Source: CAD feature listing. Evaluate the final solid. Frame: model axes, mm. Face numbers are marked on the shaded views. A direction names the side the tool comes from. Coordinates: 2 decimals unless noted, no trailing zeros. Loops run counter-clockwise (first coordinate to the right, second up) from the corner with the lowest first, then second, coordinate; pieces in that order, holes last.
Item 1: Pull-direction query (Y, two-part tool) for the marked faces 4, 5, 6 and 7; classes: +Y half, -Y half, draft (parallel to the pull), parting line (faces both ways), or undercut.
Item 2: Section query C-C, the plane z = 7. Return the cut outline in (x, y), then the cut area to 3 significant figures.
Item 3: Section query A-A, the plane x = -26.5. Return the cut outline in (y, z).
Item 4: Section query D-D, the plane x = 8. Return the cut outline in (y, z), then the cut area to 4 significant figures.
Item 5: Pin query (flat end, axial travel): pin 1 Ø3 at (x, y) = (9.5, -18.5) entering from -Z; pin 2 Ø2 at (x, y) = (28, 18.5) entering from +Z. Return the tip coordinate at first contact, or that it passes through.
Item 6: Reachability of the marked faces 1, 2 and 3 from +Z, -Z, +X, -X, +Y, -Y: full face, straight path, thin tool, end or side. Return the list, or none.
Item 7: Line query: probe 1 along Y at (x, z) = (-1.5, 12); probe 2 along X at (y, z) = (29, 7); probe 3 along X at (y, z) = (8, 6.5). Output: solid intervals per line, ascending.
Item 8: Section query B-B, the plane y = -19.5. Return the cut outline in (x, z), then the cut area to 3 significant figures.
```python
from build123d import *

# Parameters (mm, degrees)
F0_W     = 70
F0_H     = 69
F1_DEPTH = 13
F2_W     = 59.5
F2_H     = 41.5
F3_DEPTH = 8
F4_W     = 16
F4_H     = 13.75
F5_DEPTH = 13.001
F7_DEPTH = 13.001


with BuildPart() as f1:
    # F0 (on Top) → F1 (new body)
    with BuildSketch(Plane.XY):
        Rectangle(F0_W, F0_H)
    extrude(amount=F1_DEPTH)

    # F2 (on face) → F3 (cut)
    with BuildSketch(Plane.XY.offset(13)):
        Rectangle(F2_W, F2_H)
    extrude(amount=-F3_DEPTH, mode=Mode.SUBTRACT)

    # F4 (on face) → F5 (cut, through all)
    with BuildSketch(Plane.XY.offset(13)):
        with Locations((17.75, 27.625)):
            Rectangle(F4_W, F4_H)
    extrude(amount=-F5_DEPTH, mode=Mode.SUBTRACT)

    # F6 (on face) → F7 (cut, through all)
    with BuildSketch(Plane(origin=(0, 0, 0), x_dir=(1, 0, 0), z_dir=(0, 0, -1))):
        Polygon((-29.75, 15.75), (-29.75, -15.75), (-24.75, -20.75), (25.75, -20.75), (29.75, -15.75), (29.75, 15.75), (24.75, 20.75), (-24.75, 20.75), align=None)
    extrude(amount=-F7_DEPTH, mode=Mode.SUBTRACT)


solid = f1.part
```
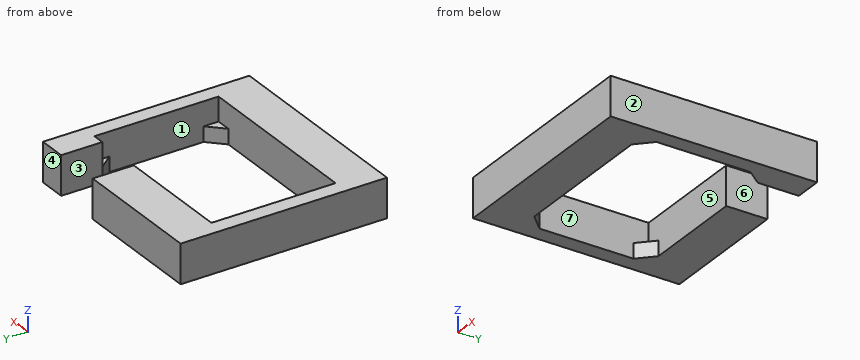
Verdict:
1. face 4: +Y half
1. face 5: undercut
1. face 6: draft
1. face 7: undercut
2. outline: (-35, -34.5) - (35, -34.5) - (35, 34.5) - (25.75, 34.5) - (25.75, 20.75) - (29.75, 20.75) - (29.75, -20.75) - (-29.75, -20.75) - (-29.75, 20.75) - (9.75, 20.75) - (9.75, 34.5) - (-35, 34.5) - close
2. area: 2,140 mm2
3. outline: (-34.5, 0) - (-19, 0) - (-19, 5) - (-20.75, 5) - (-20.75, 13) - (-34.5, 13) - close; (19, 0) - (34.5, 0) - (34.5, 13) - (20.75, 13) - (20.75, 5) - (19, 5) - close
4. outline: (-34.5, 0) - (-20.75, 0) - (-20.75, 13) - (-34.5, 13) - close; (20.75, 0) - (34.5, 0) - (34.5, 13) - (20.75, 13) - close
4. area: 357.5 mm2
5. pin 1: passes through
5. pin 2: stops at z = 5
6. face 1: +Z
6. face 2: +Z, -Z, +X, +Y, -Y
6. face 3: +Z, -Z, +Y
7. probe 1: y = -34.5 to -20.75, 20.75 to 34.5
7. probe 2: x = -35 to 9.75, 25.75 to 35
7. probe 3: x = -35 to -29.75, 29.75 to 35
8. outline: (-35, 0) - (-26, 0) - (-26, 5) - (-29.75, 5) - (-29.75, 13) - (-35, 13) - close; (26, 0) - (35, 0) - (35, 13) - (29.75, 13) - (29.75, 5) - (26, 5) - close
8. area: 174 mm2
